Here's the drawing with two shaded views (mm, measured from the low corner). I have some questions. A direction names the side the tool comes from. Round coordinates to 2 decimals unless told otherwise and drop trailing zeros. Loops run counter-clockwise (first coordinate to the right, second up) from the corner with the lowest first, then second, coordinate; pieces in that order, holes last. Notation, with made-up numbers: M -28,-10.5 L -1,-10.5 A16 ccw -1,-6.5 Z; hole C 31,-40 d2. An arc over 180 degrees is marked long. One line per item, written item: value. Start each with the question number.
Q1. Imagine slicing it at C-C (x = 5.5). Please give me the cut outline in (y, z).
Q2. I'm going to push flat-ended pins straight in: pin 1 Ø11 at (y, z) = (208, 7) entering from +X; pin 2 Ø2 at (x, y) = (19.5, 121) entering from +Z; pin 3 Ø2 at (x, z) = (31, 4.5) entering from -Y. Where does each tip first touch, or does it pass through?
Q3. Imagine slicing it at D-D (z = 18.5). Please give me the cut outline in (x, y), then the cut area to 3 significant figures.
Q4. Please list where these lines run through material, in increasing order: line 1 along X through (y, z) = (17, 33); line 2 along Y through (x, z) = (62.5, 4.5); line 3 along X through (y, z) = (197.5, 30.75).
Q5. Imagine slicing it at A-A (y = 17.5). Please give me the cut outline in (x, z).
Q6. Imagine slicing it at B-B (z = 31). Please give me the cut outline in (x, y).
Q7. Thinking about a two-plate mould opening in Z: for the marked faces 3, 4, 5 and 6, which applies, released by +Z, released by -Z, zero draft, split by the parting line, or undercut?
Q8. Which directions (+Z, -Z, +X, -X, +Y, -Y) give clear straight access to the entire face, cutting with the end or side of a thin tool? Please do the marked faces 1 and 2.
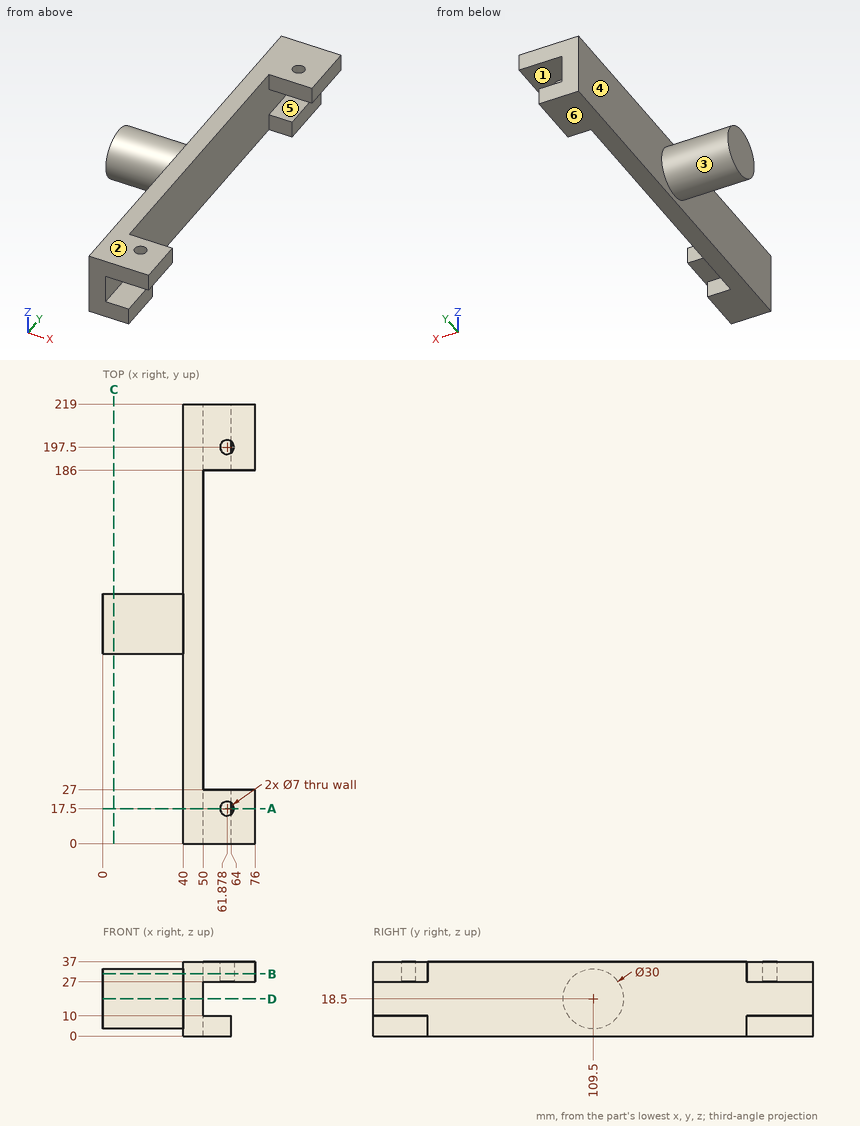
Report:
1. outline: C 109.5,18.5 d30
2. pin 1: stops at x = 64
2. pin 2: stops at z = 29.21
2. pin 3: stops at y = 102.02
3. outline: M 0,94.5 L 40,94.5 L 40,0 L 50,0 L 50,219 L 40,219 L 40,124.5 L 0,124.5 Z
3. area: 3,390 mm²
4. line 1: x = 40 to 58.41, 65.34 to 76
4. line 2: y = 0 to 27, 186 to 219
4. line 3: x = 40 to 58.38, 65.38 to 76
5. outline: M 40,0 L 64,0 L 64,10 L 50,10 L 50,27 L 58.38,27 L 58.38,37 L 40,37 Z; M 65.38,27 L 76,27 L 76,37 L 65.38,37 Z
6. outline: M 0,101.21 L 40,101.21 L 40,0 L 76,0 L 76,27 L 50,27 L 50,186 L 76,186 L 76,219 L 40,219 L 40,117.79 L 0,117.79 Z; hole C 61.88,17.5 d7; hole C 61.88,197.5 d7
7. face 3: split by the parting line
7. face 4: zero draft
7. face 5: undercut
7. face 6: released by -Z
8. face 1: +X, +Y, -Y
8. face 2: +Z, +X, -X, +Y, -Y
